Could you check a few things on this model? Use its own coordinates, in mm. Face numbers are marked on the shaded views. A direction names the side the tool comes from. Give positions to 0.01 mm unless a question says otherwise; leave off trailing zeros. Loops run counter-clockwise (first coordinate to the right, second up) from the corner with the lowest first, then second, coordinate; pieces in that order, holes last. Notation, with made-up numbers: M -2,49.25 L 5,49.25 A30 cw 5,85.25 Z; hole C 48,-1.75 d6. An arc over 180 degrees is marked long. Write each question's results on one line, items separated by ' | '. Start each with the question number.
from build123d import *

# Parameters (mm, degrees)
F0_W        = 30
F0_H        = 30
F0_R        = 3
F0_R_2      = 1.65
F0_R_3      = 2
F0_R_4      = 1.5
F1_DEPTH    = 10
F2_DEPTH    = 12
F3_DEPTH    = 4
F4_R        = 2
F5_DEPTH    = 8
F6_DEPTH    = 1
F7_DEPTH    = 4.5
F8_DEPTH    = 2
F9_DEPTH    = 2
F10_DEPTH   = 2
F11_C1_SIZE = 1.5
F11_C2_SIZE = 1.5
F11_C3_SIZE = 1.5
F11_C4_SIZE = 1.5
F11_C5_SIZE = 1.5
F12_R       = 1.65
F13_DEPTH   = 8


# Not quite as in the source:
# - a feature names something its author has since deleted; it is built from what else it names


with BuildPart() as f1:
    # F0 (on Top) → F1 (new body)
    with BuildSketch(Plane.XY):
        with Locations((15, -15)):
            Rectangle(F0_W, F0_H)
        with Locations((15, -24)):
            Circle(F0_R, mode=Mode.SUBTRACT)
        with Locations((6, -15)):
            Circle(F0_R, mode=Mode.SUBTRACT)
        with Locations((9.5, -5)):
            Circle(F0_R_2, mode=Mode.SUBTRACT)
        with Locations((15, -15)):
            Circle(F0_R_3, mode=Mode.SUBTRACT)
        with Locations((24, -15)):
            Circle(F0_R, mode=Mode.SUBTRACT)
        with Locations((15, -6)):
            Circle(F0_R, mode=Mode.SUBTRACT)
        with Locations((15, -6)):
            Circle(F0_R)
        with Locations((15, -6)):
            Circle(F0_R_4, mode=Mode.SUBTRACT)
        with Locations((15, -24)):
            Circle(F0_R)
        with Locations((15, -24)):
            Circle(F0_R_4, mode=Mode.SUBTRACT)
        with Locations((24, -15)):
            Circle(F0_R)
        with Locations((24, -15)):
            Circle(F0_R_4, mode=Mode.SUBTRACT)
        with Locations((6, -15)):
            Circle(F0_R)
        with Locations((6, -15)):
            Circle(F0_R_4, mode=Mode.SUBTRACT)
        with Locations((15, -15)):
            Circle(F0_R_3)
        with Locations((9.5, -5)):
            Circle(F0_R_2)
        with Locations((6, -15)):
            Circle(F0_R_4)
        with Locations((24, -15)):
            Circle(F0_R_4)
    extrude(amount=-F1_DEPTH)

    # F0 (on Top) → F2 (cut)
    with BuildSketch(Plane.XY):
        with Locations((15, -15)):
            Circle(F0_R_3)
    extrude(amount=-F2_DEPTH, mode=Mode.SUBTRACT)

    # F0 (on Top) → F3 (cut)
    with BuildSketch(Plane.XY):
        with Locations((15, -24)):
            Circle(F0_R)
        with Locations((15, -24)):
            Circle(F0_R_4, mode=Mode.SUBTRACT)
        with Locations((15, -6)):
            Circle(F0_R)
        with Locations((15, -6)):
            Circle(F0_R_4, mode=Mode.SUBTRACT)
    extrude(amount=-F3_DEPTH, mode=Mode.SUBTRACT)

    # F4 (on face) → F5 (cut)
    with BuildSketch(Plane(origin=(0, 0, -10), x_dir=(1, 0, 0), z_dir=(0, 0, -1))):
        with BuildLine():
            ThreePointArc((19.6, 13.0404082058), (18, 15), (19.6, 16.9595917942))
            ThreePointArc((19.6, 16.9595917942), (10, 15), (19.6, 13.0404082058))
        make_face()
        with Locations((15, 15)):
            Circle(F4_R, mode=Mode.SUBTRACT)
        with BuildLine():
            ThreePointArc((19.6, 13.0404082058), (19.8989794856, 14), (20, 15))
            ThreePointArc((20, 15), (19.8989794856, 16), (19.6, 16.9595917942))
            ThreePointArc((19.6, 16.9595917942), (18, 15), (19.6, 13.0404082058))
        make_face()
    extrude(amount=-F5_DEPTH, mode=Mode.SUBTRACT)

    # F4 (on face) → F6 (cut)
    with BuildSketch(Plane(origin=(0, 0, -10), x_dir=(1, 0, 0), z_dir=(0, 0, -1))):
        with BuildLine():
            ThreePointArc((19.6, 16.9595917942), (19.8989794856, 16), (20, 15))
            ThreePointArc((20, 15), (19.8989794856, 14), (19.6, 13.0404082058))
            ThreePointArc((19.6, 13.0404082058), (19.798982076, 13.010127694), (20, 13))
            Line((20, 13), (30, 13))
            Line((30, 13), (30, 17))
            Line((30, 17), (20, 17))
            ThreePointArc((20, 17), (19.798982076, 16.989872306), (19.6, 16.9595917942))
        make_face()
    extrude(amount=-F6_DEPTH, mode=Mode.SUBTRACT)

    # F7 (add): a face of the model
    f7_faces = [f1.faces().sort_by_distance(p)[0] for p in [
        (30, -15, -4.9391891892),
    ]]
    extrude(f7_faces, amount=F7_DEPTH)

    # F8 (add): a face of the model
    f8_faces = [f1.faces().sort_by_distance(p)[0] for p in [
        (17.25, 0, -5),
    ]]
    extrude(f8_faces, amount=F8_DEPTH)

    # F9 (add): a face of the model
    f9_faces = [f1.faces().sort_by_distance(p)[0] for p in [
        (17.25, -30, -5),
    ]]
    extrude(f9_faces, amount=F9_DEPTH)

    # F10 (add): a face of the model
    f10_faces = [f1.faces().sort_by_distance(p)[0] for p in [
        (34.5, -15, -4.9464285714),
    ]]
    extrude(f10_faces, amount=F10_DEPTH)

    # F11: chamfer of 1.5 on 6 edges, made by hand

    # F11_c1
    f11_c1_edges = [f1.edges().sort_by_distance(p)[0] for p in [
        (36.5, -5.5, -10),
    ]]
    chamfer(f11_c1_edges, length=F11_C1_SIZE)

    # F11_c2
    f11_c2_edges = [f1.edges().sort_by_distance(p)[0] for p in [
        (0, -32, -5),
    ]]
    chamfer(f11_c2_edges, length=F11_C2_SIZE)

    # F11_c3
    f11_c3_edges = [f1.edges().sort_by_distance(p)[0] for p in [
        (36.5, -32, -4.25),
    ]]
    chamfer(f11_c3_edges, length=F11_C3_SIZE)

    # F11_c4
    f11_c4_edges = [f1.edges().sort_by_distance(p)[0] for p in [
        (0, 2, -5),
    ]]
    chamfer(f11_c4_edges, length=F11_C4_SIZE)

    # F11_c5
    f11_c5_edges = [f1.edges().sort_by_distance(p)[0] for p in [
        (36.5, 2, -4.25),
    ]]
    chamfer(f11_c5_edges, length=F11_C5_SIZE)

    # F0 (on Top) + F12 (on face) → F13 (cut)
    with BuildSketch(Plane.XY):
        with Locations((9.5, -5)):
            Circle(F0_R_2)
    with BuildSketch(Plane.XY):
        with Locations((29.5, -25)):
            Circle(F12_R)
    extrude(amount=-F13_DEPTH, mode=Mode.SUBTRACT)


solid = f1.part
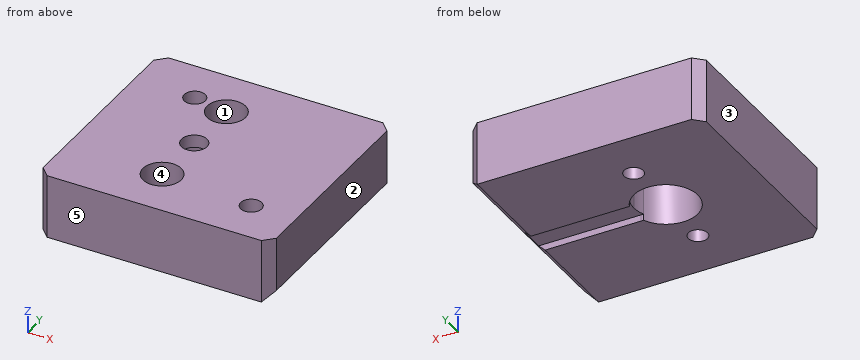
1) Which directions (+Z, -Z, +X, -X, +Y, -Y) give clear straight access to the entire face, cutting with the end or side of a thin tool? Please do the marked faces 1 and 2.
2) If we section it at C-C on y = -25: Write out the boundary of the cut face in (x, z), plus the area to 3 significant figures.
3) If we section it at B-B on z = -7: Write out the boundary of the cut face in (x, y), plus the area to 3 significant figures.
4) If we section it at A-A on x = 15: Write out the boundary of the cut face in (y, z).
5) Please list where these lines run through material, in increasing order: line 1 (Y direction, x = 15, z = -1.25); line 2 (Y direction, x = 15, z = -5.5); line 3 (X direction, y = -11, z = -3.75). Write a range as from..to.
6) If we section it at D-D on x = 29.5: Write out the boundary of the cut face in (y, z).
7) Thinking about a two-plate mould opening in X: for the marked faces 3, 4 and 5, which applies, pulls with the +X half, pulls with the -X half, needs draft (parallel to the pull), parting line crosses it, or undercut?
8) I'm going to push flat-ended pins straight in: P1, Ø3, axis at x = 29.5, y = -25, coming from the +Z side; P2, Ø4.5, axis at x = 15, y = -15, coming from the -Z side; P3, Ø5, axis at x = 15, y = -6, coming from the +Z side. Where does each tip first touch, or does it pass through?
Calculated:
1) face 1: +Z | face 2: +Z, -Z, +X, +Y, -Y
2) outline: M 0,-10 L 13.88,-10 L 13.88,-4 L 12.17,-4 L 12.17,0 L 0,0 Z; M 16.12,-10 L 35,-10 L 36.5,-8.5 L 36.5,0 L 31.15,0 L 31.15,-8 L 27.85,-8 L 27.85,0 L 17.83,0 L 17.83,-4 L 16.12,-4 Z | area: 301 mm2
3) outline: M 0,-30.5 L 1.5,-32 L 35,-32 L 36.5,-30.5 L 36.5,0.5 L 35,2 L 1.5,2 L 0,0.5 Z; hole C 9.5,-5 d3.3; hole C 15,-15 d10; hole C 15,-24 d3; hole C 15,-6 d3; hole C 29.5,-25 d3.3 | area: 1,130 mm2
4) outline: M -32,-10 L -25.5,-10 L -25.5,-4 L -27,-4 L -27,0 L -32,0 Z; M -22.5,-10 L -20,-10 L -20,-2 L -17,-2 L -17,0 L -21,0 L -21,-4 L -22.5,-4 Z; M -13,-2 L -10,-2 L -10,-10 L -7.5,-10 L -7.5,-4 L -9,-4 L -9,0 L -13,0 Z; M -4.5,-10 L 2,-10 L 2,0 L -3,0 L -3,-4 L -4.5,-4 Z
5) line 1: y = -32..-27, -21..-17, -13..-9, -3..2 | line 2: y = -32..-25.5, -22.5..-20, -10..-7.5, -4.5..2 | line 3: x = 0..12, 18..36.5
6) outline: M -32,-10 L -17,-10 L -17,-9 L -13,-9 L -13,-10 L 2,-10 L 2,0 L -23.35,0 L -23.35,-8 L -26.65,-8 L -26.65,0 L -32,0 Z
7) face 3: pulls with the -X half | face 4: undercut | face 5: needs draft
8) P1: stops at z = -8 | P2: stops at z = -2 | P3: stops at z = -4
